```python
from build123d import *

# Parameters (mm, degrees)
SKETCH2_W              = 242.645613954
SKETCH2_H              = 231.138030636
CUT_IN_HALF_DEPTH      = 165.544826719
SKETCH3_R              = 11
BALLBEARINGHOLE_DEPTH  = 165.544826719
SKETCH4_R              = 31.202879122
SUPPORTFORHOLE_DEPTH   = 4
SKETCH5_R              = 11.05
F_2NDBEARINGHOLE_DEPTH = 7
SKETCH6_R              = 4.5
INSIDEHOLE_DEPTH       = 161.277134988


with BuildPart() as part:
    # Half Circle → Sphere Revolve (revolve)
    with BuildSketch(Plane.XY):
        with BuildLine():
            Line((0, 85), (0, 95))
            ThreePointArc((0, 95), (-95, 0), (0, -95))
            Line((0, -95), (0, -85))
            ThreePointArc((0, -85), (-85, 0), (0, 85))
        make_face()
    revolve(axis=Axis((0, 85, 0), (0, 1, 0)))

    # Sketch2 → Cut in Half (cut, through all)
    with BuildSketch(Plane(origin=(0, 0, 0), x_dir=(1, 0, 0), z_dir=(0, 1, 0))):
        Rectangle(SKETCH2_W, SKETCH2_H)
    extrude(amount=-CUT_IN_HALF_DEPTH, mode=Mode.SUBTRACT)

    # Sketch3 → BallBearingHole (cut, through all)
    with BuildSketch(Plane(origin=(0, 0, 0), x_dir=(1, 0, 0), z_dir=(0, 1, 0))):
        with Locations(Location((0, 0, 0), (0, 0, 90))):
            Circle(SKETCH3_R)
    extrude(amount=BALLBEARINGHOLE_DEPTH, mode=Mode.SUBTRACT)

    # Sketch4 → SupportForHole (add)
    with BuildSketch(Plane(origin=(0, 84.4, 0), x_dir=(1, 0, 0), z_dir=(0, 1, 0))):
        Circle(SKETCH4_R)
    extrude(amount=SUPPORTFORHOLE_DEPTH)

    # Sketch5 → 2ndBearingHole (cut)
    with BuildSketch(Plane(origin=(0, 94.4, 0), x_dir=(1, 0, 0), z_dir=(0, 1, 0))):
        with Locations(Location((0, 0, 0), (0, 0, 270))):
            Circle(SKETCH5_R)
    extrude(amount=-F_2NDBEARINGHOLE_DEPTH, mode=Mode.SUBTRACT)

    # Sketch6 → InsideHole (cut, through all)
    with BuildSketch(Plane(origin=(0, 87.4, 0), x_dir=(1, 0, 0), z_dir=(0, 1, 0))):
        with Locations(Location((0, 0, 0), (0, 0, 270))):
            Circle(SKETCH6_R)
    extrude(amount=-INSIDEHOLE_DEPTH, mode=Mode.SUBTRACT)


solid = part.part
```
Could you check a few things on this model? Use its own coordinates, in mm. A direction names the side the tool comes from. Coordinates: 2 decimals unless noted, no trailing zeros. Write each loop counter-clockwise with the first axis right and the second up, starting at its lowest first coordinate (ties: lowest second). Pieces come first, ordered by that corner, then holes. Notation, with made-up numbers: (80, 54) -> (138, 54) arc R25 ccw to (138, 74) -> close; hole circle Ø3 at (38.5, 31). An arc over 180 degrees is marked (long way). Write item = value, one per line. Start each with the question number.
(1) I want a section at B-B (x = 0). Please give me the cut outline in (y, z).
(2) I need wall thicknesses on line 1 (Z direction, x = -23, y = 26.5); line 2 (Z direction, x = -8.5, y = 30); line 3 (X direction, y = 18, z = 54). Which ranges of each line are inside material? Lowest first, please. Write a range as [from, to].
(3) I want a section at C-C (y = 36). Please give me the cut outline in (x, z), plus the area to 3 significant figures.
(4) I want a section at D-D (z = 63.5). Please give me the cut outline in (x, y).
(5) We'd pull the mould along Z, two halves only. Please class faces 1 (the face through (-71, 0, 49)), 2 (the face through (1.352, 85.921, 4.292)): released by +Z, released by -Z, zero draft, split by the parting line, or undercut.
(6) Will these pins go through, and if not, where does the flat tip stop? pin 1 (20 mm diameter, centred on x = 0, z = 0, fed in from +Y); pin 2 (24 mm diameter, centred on x = 3.5, z = -3, fed in from -Y); pin 3 (10 mm diameter, centred on y = 81, z = -37, fed in from -X).
(7) I want a section at A-A (z = 0). Please give me the cut outline in (x, y), plus the area to 3 significant figures.
(8) Which directions (+Z, -Z, +X, -X, +Y, -Y) give clear straight access to the entire face, cutting with the end or side of a thin tool? Please do faces 3 (the face through (-10.787, 90.926, -2.395)), 4 (the face through (0, 84.4, 5)).
Result set:
q1.outline = (0, -95) arc R95 ccw to (94.36, -11.05) -> (87.4, -11.05) -> (87.4, -4.5) -> (84.4, -4.5) -> (84.4, -11) -> (84.29, -11) arc R85 cw to (0, -85) -> close; (0, 85) arc R85 cw to (84.29, 11) -> (84.4, 11) -> (84.4, 4.5) -> (87.4, 4.5) -> (87.4, 11.05) -> (94.36, 11.05) arc R95 ccw to (0, 95) -> close
q2.line_1 = [-88.28, -77.42], [77.42, 88.28]
q2.line_2 = [-89.74, -79.07], [79.07, 89.74]
q2.line_3 = [-76.06, -63.13], [63.13, 76.06]
q3.outline = circle Ø175.83 at (0, 0); hole circle Ø154 at (0, 0)
q3.area = 5,650 mm2
q4.outline = (-70.66, 0) -> (-56.5, 0) arc R56.5 cw to (56.5, 0) -> (70.66, 0) arc R70.66 ccw to start
q5.face_1 = zero draft
q5.face_2 = undercut
q6.pin_1 = 87.4
q6.pin_2 = 83.36
q6.pin_3 = -44.28
q7.outline = (-95, 0) -> (-85, 0) arc R85 cw to (-11, 84.29) -> (-11, 84.4) -> (-4.5, 84.4) -> (-4.5, 87.4) -> (-11.05, 87.4) -> (-11.05, 94.36) arc R95 ccw to start; (4.5, 84.4) -> (11, 84.4) -> (11, 84.29) arc R85 cw to (85, 0) -> (95, 0) arc R95 ccw to (11.05, 94.36) -> (11.05, 87.4) -> (4.5, 87.4) -> close
q7.area = 2,650 mm2
q8.face_3 = +Y
q8.face_4 = -Y
